```python
from build123d import *

# Parameters (mm, degrees)
F1_DEPTH = 12.7
F2_DEPTH = 129.54
F3_R     = 20.726602
F4_DEPTH = 217.424


with BuildPart() as f1:
    # F0 (on Front) → F1 (new body, symmetric)
    with BuildSketch(Plane.XZ):
        Polygon((-76.2, 25.4), (-76.2, 0), (0, 0), (0, 152.4), (-25.4, 152.4), (-25.4, 25.4), align=None)
    extrude(amount=F1_DEPTH, both=True)

    # F1_face (on face) → F2 (join)
    with BuildSketch(Plane(origin=(-22.225, -12.7, 60.325), x_dir=(1, 0, 0), z_dir=(0, -1, 0))):
        Polygon((-53.975, -34.925), (-53.975, -60.325), (22.225, -60.325), (22.225, 92.075), (-3.175, 92.075), (-3.175, -34.925), align=None)
    extrude(amount=-F2_DEPTH)

    # F3 (on face) → F4 (cut, symmetric)
    with BuildSketch(Plane(origin=(-25.4, 0, 0), x_dir=(0, -1, 0), z_dir=(-1, 0, 0))):
        with Locations((-44.110455, 117.932089)):
            Circle(F3_R)
    extrude(amount=F4_DEPTH, both=True, mode=Mode.SUBTRACT)


solid = f1.part
```
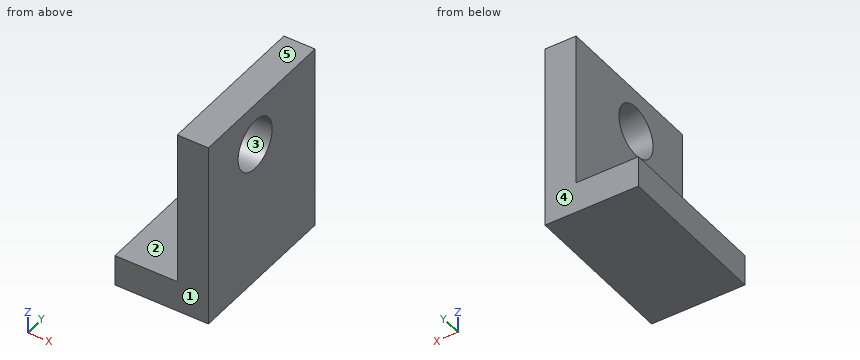
Model file for the job. Use its own axes, mm. Face numbers are marked on the shaded views. A direction names the side the tool comes from. Round coordinates to 2 decimals unless told otherwise and drop trailing zeros. Write each loop counter-clockwise with the first axis right and the second up, starting at its lowest first coordinate (ties: lowest second). Pieces come first, ordered by that corner, then holes. Notation, with made-up numbers: (-9.75, 75.25) - (11.25, 75.25) arc R18 ccw to (11.25, 82.25) - close; hole circle Ø3 at (77.25, 86.5). An arc over 180 degrees is marked (long way). One line per item, written item: value.
(1) 3-axis set-ups, long thin cutter, end or side, ignore diameter. For the marked faces 1 and 2: which of +Z, -Z, +X, -X, +Y, -Y reach the whole face in a straight line?
Values follow:
face 1: +Z, -Z, +X, -X, -Y
face 2: +Z, -X, +Y, -Y
(2) Cut at D-D, the plane x = -5.5. Give the cut face in (y, z).
Values follow:
outline: (-12.7, 0) - (116.84, 0) - (116.84, 152.4) - (-12.7, 152.4) - close; hole circle Ø41.45 at (44.11, 117.93)
(3) Drop flat-ended pins along their axis: P1, Ø8, axis at y = 19.5, z = 57.5, coming from the -X side; P2, Ø8, axis at x = -31.5, y = 5, coming from the +Z side. Give the stop position or say it passes through.
Values follow:
P1: stops at x = -25.4
P2: stops at z = 25.4
(4) Wall check: probe 1 along Z at (x, y) = (-20, 45); probe 2 along X at (y, z) = (85, 54); probe 3 along Z at (x, y) = (-52, 3). Give the ranges that are in metal, low to high.
Values follow:
probe 1: z = 0 to 97.22, 138.64 to 152.4
probe 2: x = -25.4 to 0
probe 3: z = 0 to 25.4
(5) Two-plate mould, pull along Y, no slides. Class the marked faces 3, 4 and 5: pulls with the +Y half, pulls with the -Y half, needs draft (parallel to the pull), parting line crosses it, or undercut.
Values follow:
face 3: undercut
face 4: pulls with the +Y half
face 5: needs draft
(6) Cut at C-C, the plane y = 76. Give the cut face in (x, z), plus the area to 3 significant figures.
Values follow:
outline: (-76.2, 0) - (0, 0) - (0, 152.4) - (-25.4, 152.4) - (-25.4, 25.4) - (-76.2, 25.4) - close
area: 5,160 mm²
(7) Cut at A-A, the plane y = 49. Give the cut face in (x, z), plus the area to 3 significant figures.
Values follow:
outline: (-76.2, 0) - (0, 0) - (0, 97.79) - (-25.4, 97.79) - (-25.4, 25.4) - (-76.2, 25.4) - close; (-25.4, 138.07) - (0, 138.07) - (0, 152.4) - (-25.4, 152.4) - close
area: 4,140 mm²
(8) Cut at B-B, the plane z = 131. Give the cut face in (x, y).
Values follow:
outline: (-25.4, -12.7) - (0, -12.7) - (0, 28.02) - (-25.4, 28.02) - close; (-25.4, 60.2) - (0, 60.2) - (0, 116.84) - (-25.4, 116.84) - close
